Verification items for this drawing (mm, ordinates from the low corner). Round coordinates to 2 decimals unless told otherwise and drop trailing zeros. Order: outer loops, then holes, each group sorted by start corner. A loop starts at its lowest first (then second) coordinate and runs counter-clockwise, first axis right, second up.
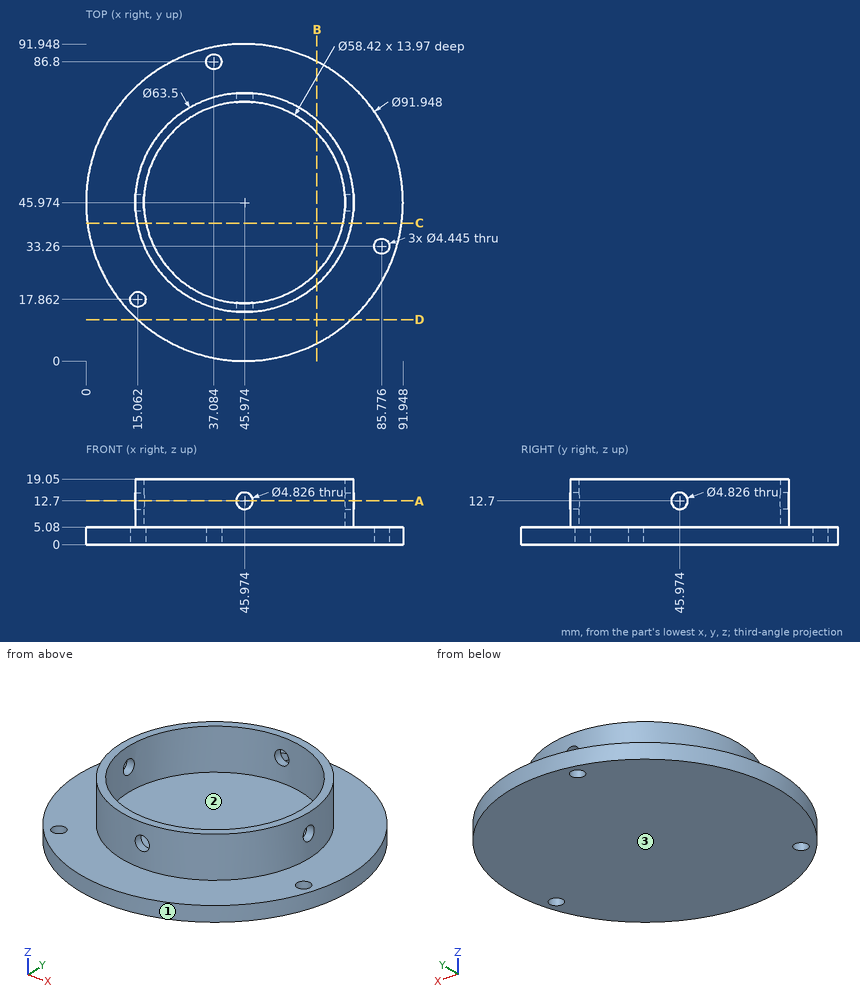
Item 1: Sectioned sample at A-A (z = 12.7). Record the cut outline in (x, y).
Answer:
outline: (14.32, 43.56) arc R31.75 ccw to (43.56, 14.32) - (43.56, 16.86) arc R29.21 cw to (16.86, 43.56) - close; (14.32, 48.39) - (16.86, 48.39) arc R29.21 cw to (43.56, 75.08) - (43.56, 77.63) arc R31.75 ccw to start; (48.39, 14.32) arc R31.75 ccw to (77.63, 43.56) - (75.08, 43.56) arc R29.21 cw to (48.39, 16.86) - close; (48.39, 75.08) arc R29.21 cw to (75.08, 48.39) - (77.63, 48.39) arc R31.75 ccw to (48.39, 77.63) - close
Item 2: Scan lines: line 1 along Y through (x, z) = (45.5, 16.5); line 2 along Z through (x, y) = (11, 51.5); line 3 along X through (y, z) = (44, 18) (1 decimal). Record each from-to range of solid material in increasing order.
Answer:
line 1: y = 14.23 to 16.77, 75.18 to 77.72
line 2: z = 0 to 5.08
line 3: x = 14.3 to 16.8, 75.1 to 77.7
Item 3: Sectioned sample at C-C (y = 40). Record the cut outline in (x, z).
Answer:
outline: (0.39, 0) - (91.56, 0) - (91.56, 5.08) - (77.16, 5.08) - (77.16, 19.05) - (74.57, 19.05) - (74.57, 5.08) - (17.38, 5.08) - (17.38, 19.05) - (14.79, 19.05) - (14.79, 5.08) - (0.39, 5.08) - close
Item 4: Sectioned sample at D-D (y = 12). Record the cut outline in (x, z).
Answer:
outline: (15, 0) - (76.95, 0) - (76.95, 5.08) - (15, 5.08) - close
Item 5: Release check for a two-part mould opening along Y. For the marked faces 1, 2 and 3 record: released by +Y, released by -Y, zero draft, split by the parting line, or undercut.
Answer:
face 1: split by the parting line
face 2: undercut
face 3: zero draft
Item 6: Go/stop test with flat-tipped pins: P1, Ø4, axis at y = 45.974, z = 12.7, coming from the +X side; P2, Ø5, axis at y = 75.5, z = 15.5, coming from the +X side (1 decimal); P3, Ø5, axis at x = 85.78, y = 33.26, coming from the +Z side; P4, Ø8, axis at x = 51, z = 6, coming from the +Y side. Record where each tip stops, or that it passes through.
Answer:
P1: passes through
P2: stops at x = 62.6
P3: stops at z = 5.08
P4: stops at y = 91.93
Item 7: Sectioned sample at B-B (x = 67). Record the cut outline in (y, z).
Answer:
outline: (5.09, 0) - (86.86, 0) - (86.86, 5.08) - (69.76, 5.08) - (69.76, 19.05) - (66.25, 19.05) - (66.25, 5.08) - (25.7, 5.08) - (25.7, 19.05) - (22.18, 19.05) - (22.18, 5.08) - (5.09, 5.08) - close
